Check sheet for the drawn part. Datum: minimum x, y, z corner. Units: mm. Round coordinates to 2 decimals unless told otherwise and drop trailing zeros. Loops run counter-clockwise (first coordinate to the right, second up) from the corner with the lowest first, then second, coordinate; pieces in that order, holes last.
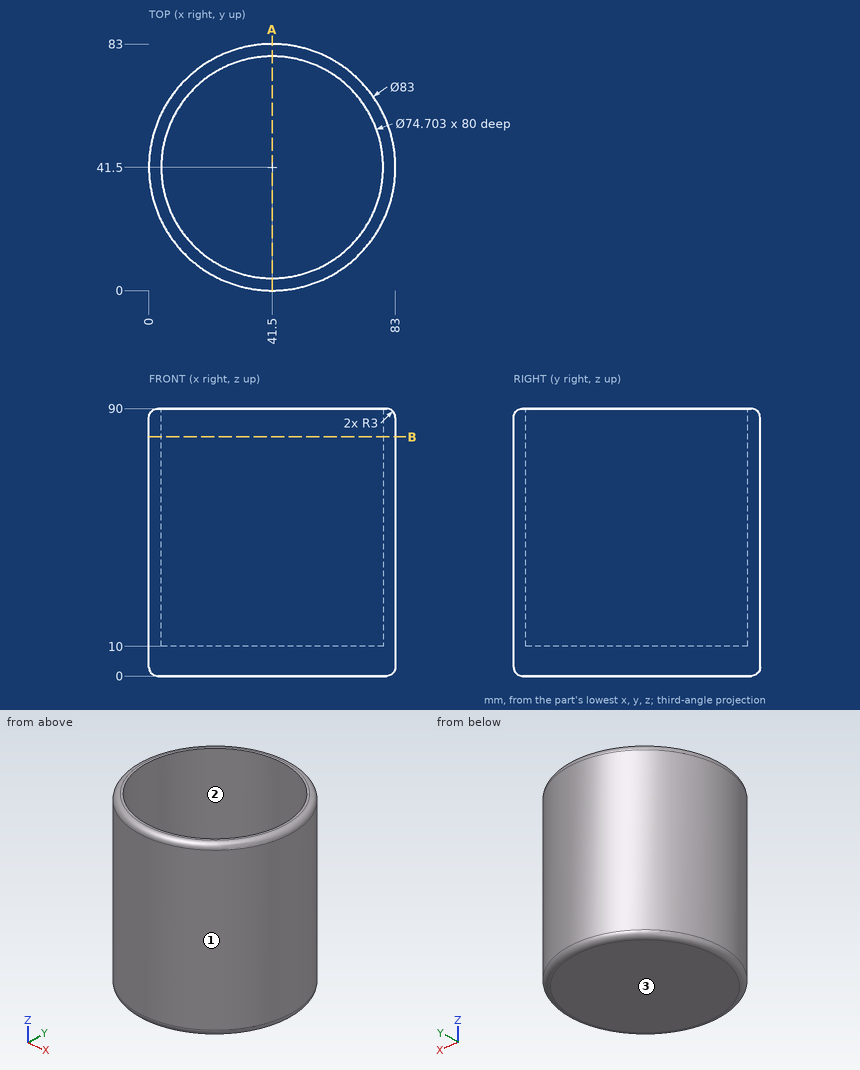
1) Scan lines: line 1 along Y through (x, z) = (41, 59); line 2 along Y through (x, z) = (25, 60.5). Record each from-to range of solid material in increasing order.
Report:
line 1: y = 0 to 4.15, 78.85 to 83
line 2: y = 3.42 to 7.99, 75.01 to 79.58
2) Mould release check, pull along X, two halves, no side actions. Record for the marked faces 1, 2 and 3: +X half, -X half, draft (parallel to the pull), parting line (faces both ways), or undercut.
Report:
face 1: parting line
face 2: undercut
face 3: draft
3) Sectioned sample at B-B, the plane z = 80.5. Record the cut outline in (x, y).
Report:
outline: circle Ø83 at (41.5, 41.5); hole circle Ø74.7 at (41.5, 41.5)
4) Gauge pin test, flat ends, axial feed: pin 1 (10 mm diameter, centred on x = 31.5, z = 15, fed in from +Y); pin 2 (1 mm diameter, centred on y = 29, z = 11.5, fed in from +X); pin 3 (6 mm diameter, centred on x = 30.5, z = 22, fed in from -Y). Record the tip position at first contact, or that the pin passes through.
Report:
pin 1: stops at y = 82.7
pin 2: stops at x = 81.23
pin 3: stops at y = 0.78
5) Sectioned sample at A-A, the plane x = 41.5. Record the cut outline in (y, z).
Report:
outline: (0, 3) arc R3 ccw to (3, 0) - (80, 0) arc R3 ccw to (83, 3) - (83, 87) arc R3 ccw to (80, 90) - (78.85, 90) - (78.85, 10) - (4.15, 10) - (4.15, 90) - (3, 90) arc R3 ccw to (0, 87) - close
